Autodesk Inventor part; units mm, degrees
ref_plane "Start Plane" through (0, 0, -25) normal (0, 0, 1) x (1, 0, 0)
ref_plane "End Plane" through (0, 0, 835.0026) normal (0, 0, 1) x (1, 0, 0)
ref_plane "Work Plane4" through (25, 0, 835.0026) normal (-0.7071, 0, 0.7071) x (0.7071, 0, 0.7071)
ref_plane "Start Plane" through (0, 0, -25) normal (0, 0, 1) x (1, 0, 0)
ref_plane "End Plane" through (0, 0, 835.0026) normal (0, 0, 1) x (1, 0, 0)
sketch "Sketch" plane through (0, 0, 0) normal (0, 0, 1) x (1, 0, 0)
  line L0 (-25, -21) -> (-25, 21)
  line L1 (-21, 25) -> (21, 25)
  line L2 (25, 21) -> (25, -21)
  line L3 (21, -25) -> (-21, -25)
  arc A0 (-25, -21) -> (-21, -25) centre (-21, -21) ccw
  arc A1 (25, 21) -> (21, 25) centre (21, 21) ccw
  arc A2 (-21, 25) -> (-25, 21) centre (-21, 21) ccw
  arc A3 (21, -25) -> (25, -21) centre (21, -21) ccw
  arc A4 (-21, 23) -> (-23, 21) centre (-21, 21) ccw
  line L4 (-21, 23) -> (21, 23)
  arc A5 (23, 21) -> (21, 23) centre (21, 21) ccw
  line L5 (23, 21) -> (23, -21)
  arc A6 (21, -23) -> (23, -21) centre (21, -21) ccw
  line L6 (21, -23) -> (-21, -23)
  arc A7 (-23, -21) -> (-21, -23) centre (-21, -21) ccw
  line L7 (-23, -21) -> (-23, 21)
  line L8 (0, 36.1598) -> (0, -36.1598) construction
  line L9 (-36.1598, 0) -> (36.1598, 0) construction
  dimension "d7" = 4
  dimension "d9" = 50
  dimension "d11" = 50
  dimension "d12" = 2
  dimension "d15" = 25
  dimension "d16" = 25
extrude "Body" add sketch "Sketch" along normal up to surface (860.0026 mm away) from surface at -25
sketch "Sketch3" plane through (0, 0, 0) normal (0, 0, 1) x (1, 0, 0)
  line L0 (0, 0) -> (10, 0)
ref_plane "Work Plane3" through (0, 0, 0) normal (0, -1, 0) x (1, 0, 0)
sketch "Sketch4" plane through (0, 0, 0) normal (0, -1, 0) x (1, 0, 0)
  line L0 (-2, -25) -> (12, -25)
  line L1 (-2, 835.0026) -> (12, 835.0026)
  dimension "d18" = 860.0026
ref_plane "Work Plane4" through (25, 0, 835.0026) normal (-0.7071, 0, 0.7071) x (0.7071, 0, 0.7071)
split "Split1" plane through (25, 0, 835.0026) removes the side toward (-0.7071, 0, 0.7071)
ref_plane "Work Plane5" through (25, 0, -25) normal (-0.7071, 0, -0.7071) x (-0.7071, 0, 0.7071)
split "Split2" plane through (25, 0, -25) removes the side toward (-0.7071, 0, -0.7071)
sketch "Sketch5" plane through (25, -21, 835.0026) normal (1, 0, 0) x (0, 0, -1)
  circle A0 centre (554, 21) radius 6
  circle A1 centre (414, 21) radius 6
  circle A2 centre (190, 21) radius 8
  circle A3 centre (70, 21) radius 8
  point P0 (835.0026, 21)
extrude "Extrusion2" cut sketch "Sketch5" against normal up to surface (50 mm away)
equation "\"d7\" = G_IR"
equation "\"d9\" = G_W"
equation "\"d11\" = G_H"
equation "\"d12\" = G_T"
equation "\"d15\" = 0.5 * d9"
equation "\"d16\" = 0.5 * d11"
equation "\"d3\" = G_L"
equation "\"G_W\" = 50"
equation "\"G_H\" = 50"
equation "\"G_T\" = 2"
equation "\"G_IR\" = 4"
equation "\"G_L\" = d18"
equation "\"G_OFFSET_START\" = 25"
equation "\"G_OFFSET_END\" = 25"
equation "\"d13\" = -G_OFFSET_START"
equation "\"d14\" = G_OFFSET_END + B_L"
equation "\"B_L\" = 810.0026"
properties part number "ISO 10799-2 - 50x50x2 - 860"
Part model, mm, in its own coordinate system. A direction names the side the tool comes from. Coordinates: 2 decimals unless noted, no trailing zeros. Order: outer loops, then holes, each group sorted by start corner. A loop starts at its lowest first (then second) coordinate and runs counter-clockwise, first axis right, second up. Notation, with made-up numbers: (26.25, 63) - (66.25, 63) arc R28 ccw to (66.25, 86) - close; hole circle Ø10 at (79.25, 55). An arc over 180 degrees is marked (long way). Return JSON: item names as keys, results as strings. Group by question number.
Item 1: Which spindle directions (+Z, -Z, +X, -X, +Y, -Y) get a long thin tool onto all of the face, cutting with end or side? Do faces 4 (the face through (-2, 24, 2)), 5 (the face through (0, -23, 399)). Say none if no direction does.
Item 2: Pin check, flat tip, straight feed: pin 1 (21 mm diameter, centred on y = 0, z = 645, fed in from -X). Stop position of the tip, or through.
Item 3: Drill centre lines: probe 1 along X at (y, z) = (12, 346.5); probe 2 along Y at (x, z) = (22.5, 422.5). Where is each one in solid material? Low to high. Write a range as from..to.
Item 4: Pull direction Y, two halves, no side cores. Call faces 1 (the face through (0, -25, 399)), 2 (the face through (0, 25, 399)), 3 (the face through (-23.986, 0.352, 772.995)): pulls with the +Y half, pulls with the -Y half, needs draft (parallel to the pull), parting line crosses it, or undercut.
Item 5: Cut at B-B (z = 301). List the corners of the cut face in (x, y), plus the area to 3 significant figures.
Item 6: Cut at A-A (x = 11.5). List the corners of the cut face in (y, z), plus the area to 3 significant figures.
Check values:
{
 "1": {"face 4": "-Z, -X, +Y, -Y", "face 5": "+Z, -Z"},
 "2": {"pin 1": "stops at x = -25"},
 "3": {"probe 1": "x = -25..-23, 23..25", "probe 2": "y = -24.71..-22.32, 22.32..24.71"},
 "4": {"face 1": "pulls with the -Y half", "face 2": "pulls with the +Y half", "face 3": "undercut"},
 "5": {"outline": "(-25, -21) arc R4 ccw to (-21, -25) - (21, -25) arc R4 ccw to (25, -21) - (25, 21) arc R4 ccw to (21, 25) - (-21, 25) arc R4 ccw to (-25, 21) - close; hole (-23, -21) arc R2 ccw to (-21, -23) - (21, -23) arc R2 ccw to (23, -21) - (23, 21) arc R2 ccw to (21, 23) - (-21, 23) arc R2 ccw to (-23, 21) - close", "area": "374 mm2"},
 "6": {"outline": "(-25, -11.5) - (-23, -11.5) - (-23, 821.5) - (-25, 821.5) - close; (23, -11.5) - (25, -11.5) - (25, 821.5) - (23, 821.5) - close", "area": "3,330 mm2"}
}
